```python
from build123d import *

# Parameters (mm, degrees)
F0_W     = 38.1
F0_H     = 279.4
F1_DEPTH = 6.35
F2_W     = 25.4
F2_H     = 6.35
F4_DEPTH = 6.35
F3_W     = 25.4
F3_H     = 6.35
F5_DEPTH = 6.35


with BuildPart() as f1:
    # F0 (on Top) → F1 (new body)
    with BuildSketch(Plane.XY):
        with Locations((19.05, 139.7)):
            Rectangle(F0_W, F0_H)
    extrude(amount=F1_DEPTH)

    # F2 (on face) → F4 (join)
    with BuildSketch(Plane.YZ.offset(38.1)):
        with Locations((241.3, 3.175)):
            Rectangle(F2_W, F2_H)
        with Locations((190.5, 3.175)):
            Rectangle(F2_W, F2_H)
        with Locations((139.7, 3.175)):
            Rectangle(F2_W, F2_H)
        with Locations((88.9, 3.175)):
            Rectangle(F2_W, F2_H)
        with Locations((38.1, 3.175)):
            Rectangle(F2_W, F2_H)
    extrude(amount=F4_DEPTH)

    # F3 (on face) → F5 (join)
    with BuildSketch(Plane(origin=(0, 0, 0), x_dir=(0, -1, 0), z_dir=(-1, 0, 0))):
        with Locations((-38.1, 3.175)):
            Rectangle(F3_W, F3_H)
        with Locations((-88.9, 3.175)):
            Rectangle(F3_W, F3_H)
        with Locations((-139.7, 3.175)):
            Rectangle(F3_W, F3_H)
        with Locations((-190.5, 3.175)):
            Rectangle(F3_W, F3_H)
        with Locations((-241.3, 3.175)):
            Rectangle(F3_W, F3_H)
    extrude(amount=F5_DEPTH)


solid = f1.part
```
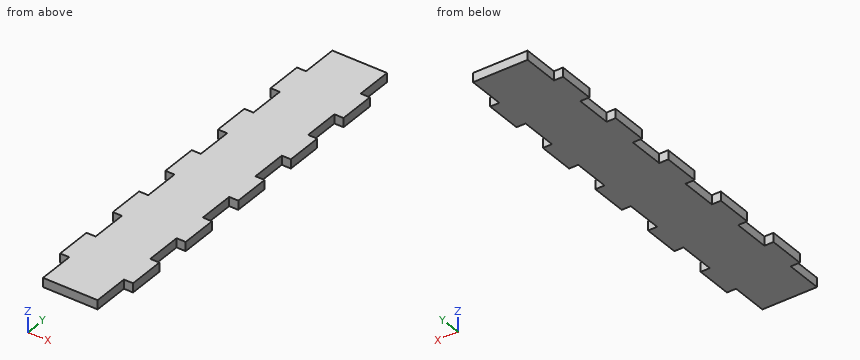
Part model, mm, in its own coordinate system. Round coordinates to 2 decimals unless told otherwise and drop trailing zeros. Write each loop counter-clockwise with the first axis right and the second up, starting at its lowest first coordinate (ties: lowest second). Pieces come first, ordered by that corner, then holes.
Item 1: Drop flat-ended pins along their axis: pin 1 Ø3 at (y, z) = (15.5, 3) entering from +X; pin 2 Ø3 at (x, z) = (-3.5, 2) entering from -Y; pin 3 Ø1 at (y, z) = (221.5, 2.5) entering from -X. Give the stop position or say it passes through.
Results:
pin 1: stops at x = 38.1
pin 2: stops at y = 25.4
pin 3: stops at x = 0
Item 2: Probe L1, parallel to Y at x = -4, z = 2.5; L2, parallel to X at y = 120, z = 4. List the from-to ranges inside material, lowest first.
Results:
L1: y = 25.4 to 50.8, 76.2 to 101.6, 127 to 152.4, 177.8 to 203.2, 228.6 to 254
L2: x = 0 to 38.1
Item 3: Cut at A-A, the plane y = 162. Give the cut face in (x, z), plus the area to 3 significant figures.
Results:
outline: (0, 0) - (38.1, 0) - (38.1, 6.35) - (0, 6.35) - close
area: 242 mm2
